Input: part model. Units: mm. Frame: model coordinates. A direction names the side the tool comes from. Coordinates: 2 decimals unless noted, no trailing zeros. Order: outer loops, then holes, each group sorted by start corner. A loop starts at its lowest first (then second) coordinate and runs counter-clockwise, first axis right, second up. Notation, with made-up numbers: (-19.75, -7.5) -> (1.25, -7.5) arc R30 cw to (1.25, 25.5) -> close; hole circle Ø1 at (-30, 80). An arc over 180 degrees is marked (long way). Answer as CSV lines item,"result".
from build123d import *

# Parameters (mm, degrees)
F0_W            = 116
F0_H            = 56
F0_W_2          = 104
F0_H_2          = 44
F1_DEPTH        = 20
F2_W            = 110
F2_H            = 50
F2_W_2          = 104
F2_H_2          = 44
F3_DEPTH        = 3
F4_W            = 4
F4_H            = 20
F5_DEPTH        = 34
F6_W            = 3.5
F6_H            = 20
F7_DEPTH        = 15
F8_W            = 3.5
F8_H            = 20
F9_DEPTH        = 15
F11_D           = 3.3
F11_DEPTH       = 5
F11_CSINK_D     = 6.72
F11_CSINK_ANGLE = 90
F11_TIP         = 0.9914200214
F13_D           = 3.3
F13_DEPTH       = 5
F13_CSINK_D     = 6.72
F13_CSINK_ANGLE = 90
F13_TIP         = 0.9914200214
F14_R           = 3


with BuildPart() as f1:
    # F0 (on Top) → F1 (new body)
    with BuildSketch(Plane.XY):
        Rectangle(F0_W, F0_H)
        Rectangle(F0_W_2, F0_H_2, mode=Mode.SUBTRACT)
    extrude(amount=F1_DEPTH)

    # F2 (on face) → F3 (cut)
    with BuildSketch(Plane.XY.offset(20)):
        Rectangle(F2_W, F2_H)
        Rectangle(F2_W_2, F2_H_2, mode=Mode.SUBTRACT)
    extrude(amount=-F3_DEPTH, mode=Mode.SUBTRACT)

    # F4 (on face) → F5 (join)
    with BuildSketch(Plane.XZ.offset(28)):
        with Locations((-56, 10)):
            Rectangle(F4_W, F4_H)
        with Locations((56, 10)):
            Rectangle(F4_W, F4_H)
    extrude(amount=F5_DEPTH)

    # F6 (on face) → F7 (join)
    with BuildSketch(Plane.YZ.offset(58)):
        with Locations((-60.25, 10)):
            Rectangle(F6_W, F6_H)
    extrude(amount=F7_DEPTH)

    # F8 (on face) → F9 (join)
    with BuildSketch(Plane(origin=(-58, 0, 0), x_dir=(0, -1, 0), z_dir=(-1, 0, 0))):
        with Locations((60.25, 10)):
            Rectangle(F8_W, F8_H)
    extrude(amount=F9_DEPTH)

    # F11
    with Locations(Plane(origin=(0, -58.5, 0), x_dir=(-1, 0, 0), z_dir=(0, 1, 0))):
        with Locations((-65.5, 10)):
            CounterSinkHole(F11_D / 2, F11_CSINK_D / 2, depth=F11_DEPTH, counter_sink_angle=F11_CSINK_ANGLE)
            with Locations((0, 0, -(F11_DEPTH + F11_TIP / 2))):  # 118° drill point
                Cone(0, F11_D / 2, F11_TIP, mode=Mode.SUBTRACT)

    # F13
    with Locations(Plane(origin=(0, -58.5, 0), x_dir=(-1, 0, 0), z_dir=(0, 1, 0))):
        with Locations((65.5, 10)):
            CounterSinkHole(F13_D / 2, F13_CSINK_D / 2, depth=F13_DEPTH, counter_sink_angle=F13_CSINK_ANGLE)
            with Locations((0, 0, -(F13_DEPTH + F13_TIP / 2))):  # 118° drill point
                Cone(0, F13_D / 2, F13_TIP, mode=Mode.SUBTRACT)

    # F14
    f14_edges = [f1.edges().sort_by_distance(p)[0] for p in [
        (58, 28, 10),
        (-58, 28, 10),
        (73, -60.25, 0),
        (73, -60.25, 20),
        (-73, -60.25, 20),
        (-73, -60.25, 0),
    ]]
    fillet(f14_edges, radius=F14_R)


solid = f1.part
1. Mould query, pull axis Y, two halves, no side actions, for faces 6 (the face through (-72.14, -60.27, 0.9)), 7 (the face through (-55, 0, 19)), 8 (the face through (57.14, 27.1, 10.14)). Classes: released by +Y, released by -Y, zero draft, split by the parting line, or undercut.
Findings:
face 6,"zero draft"
face 7,"undercut"
face 8,"released by +Y"
2. Contact query for flat-ended pins moving along their axis: pin 1 (6 mm diameter, centred on x = -19.5, z = 12.5, fed in from -Y); pin 2 (5 mm diameter, centred on y = -7.5, z = 12.5, fed in from -X); pin 3 (5 mm diameter, centred on y = -8, z = 11, fed in from +X). Output: stop coordinate, or through.
Findings:
pin 1,"stops at y = -28"
pin 2,"stops at x = -58"
pin 3,"stops at x = 58"
3. Ray query, line 1 along X through (y, z) = (-61.35, 10); line 2 along Y through (x, z) = (-34, 13); line 3 along X through (y, z) = (10.5, 16.75). Return the intervals inside material, ascending.
Findings:
line 1,"x = -73 to -67.15, -63.85 to -54, 54 to 63.85, 67.15 to 73"
line 2,"y = -28 to -22, 22 to 28"
line 3,"x = -58 to -52, 52 to 58"
4. Cut plane C-C (y = -43). Return the cut outline in (x, z), plus the area to 3 significant figures.
Findings:
outline,"(-58, 0) -> (-54, 0) -> (-54, 20) -> (-58, 20) -> close; (54, 0) -> (58, 0) -> (58, 20) -> (54, 20) -> close"
area,"160 mm2"
5. Cut plane B-B (x = 34.5). Return the cut outline in (y, z).
Findings:
outline,"(-28, 0) -> (-22, 0) -> (-22, 17) -> (-25, 17) -> (-25, 20) -> (-28, 20) -> close; (22, 0) -> (28, 0) -> (28, 20) -> (25, 20) -> (25, 17) -> (22, 17) -> close"
6. Cut plane D-D (x = -65.5). Return the cut outline in (y, z).
Findings:
outline,"(-62, 0) -> (-58.5, 0) -> (-58.5, 6.64) -> (-60.21, 8.35) -> (-62, 8.35) -> close; (-62, 11.65) -> (-60.21, 11.65) -> (-58.5, 13.36) -> (-58.5, 20) -> (-62, 20) -> close"
7. Reachability of faces 1 (the face through (62, -58.5, 12)), 2 (the face through (55, 0, 19)), 3 (the face through (-62, -58.5, 12)), 4 (the face through (-54, -45, 10)), 5 (the face through (-1, 22, 8)) from +Z, -Z, +X, -X, +Y, -Y: full face, straight path, thin tool, end or side. Return the list, or none.
Findings:
face 1,"+Z, -Z, +X, +Y"
face 2,"+Z"
face 3,"+Z, -Z, -X, +Y"
face 4,"+Z, -Z, -Y"
face 5,"+Z, -Z"
8. Cut plane A-A (z = 10). State how many separate pieces and enclosed holes the cut face has, plus the area to 3 significant figures.
Findings:
separate pieces,"3"
enclosed holes,"1"
area,"2,260 mm2"
